Design review of the part built by this model. Coordinates are the model's own, in mm. Face numbers are marked on the shaded views. A direction names the side the tool comes from. Coordinates: 2 decimals unless noted, no trailing zeros. Loops run counter-clockwise (first coordinate to the right, second up) from the corner with the lowest first, then second, coordinate; pieces in that order, holes last. Notation, with made-up numbers: M -39.5,15.5 L -7.5,15.5 A20 cw -7.5,39.5 Z; hole C 26.5,44.5 d11. An arc over 180 degrees is marked long. One line per item, written item: value.
```python
from build123d import *

# Parameters (mm, degrees)
F1_DEPTH  = 25
F3_DEPTH  = 3.96875
F4_R      = 3.81
F5_DEPTH  = 21.001
F6_R      = 7.5
F7_DEPTH  = 2
F8_R      = 26.5
F8_R_2    = 21.5
F9_DEPTH  = 25
F10_W     = 41.7897145033
F10_H     = 10
F11_DEPTH = 26.501
F12_R     = 5
F13_R     = 12


# Not quite as in the source:
# - a length typed as a fraction of an inch, garbled in the dataset ("3 / 203.2 mm" for 3/8 in), is restored


with BuildPart() as f1:
    # F0 (on Right) → F1 (new body, symmetric)
    with BuildSketch(Plane.YZ):
        with BuildLine():
            Line((-24.2330926563, 5), (-9.2330926563, 5))
            ThreePointArc((-9.2330926563, 5), (-5.3735463151, 9.0208092763), (0, 10.5))
            Line((0, 10.5), (-24.2330926563, 10.5))
            Line((-24.2330926563, 10.5), (-24.2330926563, 5))
        make_face()
        with BuildLine():
            ThreePointArc((-2.2912878475, 5), (2.9705148408, 4.628827236), (5.5, 0))
            ThreePointArc((5.5, 0), (2.9705148408, -4.628827236), (-2.2912878475, -5))
            Line((-2.2912878475, -5), (-9.2330926563, -5))
            ThreePointArc((-9.2330926563, -5), (-5.3735463151, -9.0208092763), (0, -10.5))
            ThreePointArc((0, -10.5), (7.4246212025, -7.4246212025), (10.5, 0))
            ThreePointArc((10.5, 0), (7.4246212025, 7.4246212025), (0, 10.5))
            ThreePointArc((0, 10.5), (-5.3735463151, 9.0208092763), (-9.2330926563, 5))
            Line((-9.2330926563, 5), (-2.2912878475, 5))
        make_face()
        with BuildLine():
            ThreePointArc((0, -10.5), (-5.3735463151, -9.0208092763), (-9.2330926563, -5))
            Line((-9.2330926563, -5), (-24.2330926563, -5))
            Line((-24.2330926563, -5), (-24.2330926563, -10.5))
            Line((-24.2330926563, -10.5), (0, -10.5))
        make_face()
    extrude(amount=F1_DEPTH, both=True)

    # F2 (on face) → F3 (cut)
    with BuildSketch(Plane(origin=(0, 0, -10.5), x_dir=(1, 0, 0), z_dir=(0, 0, -1))):
        Polygon((19.1395280957, 12.1165463282), (15.8197640478, 17.8665463282), (9.1802359522, 17.8665463282), (5.8604719043, 12.1165463282), (9.1802359522, 6.3665463282), (15.8197640478, 6.3665463282), align=None)
        Polygon((-15.8197640478, 6.3665463282), (-9.1802359522, 6.3665463282), (-5.8604719043, 12.1165463282), (-9.1802359522, 17.8665463282), (-15.8197640478, 17.8665463282), (-19.1395280957, 12.1165463282), align=None)
    extrude(amount=-F3_DEPTH, mode=Mode.SUBTRACT)

    # F4 (on face) → F5 (cut, through all)
    with BuildSketch(Plane(origin=(0, 0, -10.5), x_dir=(1, 0, 0), z_dir=(0, 0, -1))):
        with Locations((12.5, 12.1165463282)):
            Circle(F4_R)
        with Locations((-12.5, 12.1165463282)):
            Circle(F4_R)
    extrude(amount=-F5_DEPTH, mode=Mode.SUBTRACT)

    # F6 (on face) → F7 (cut)
    with BuildSketch(Plane.XY.offset(10.5)):
        with Locations((-12.5, -12.1165463282)):
            Circle(F6_R)
        with Locations((12.5, -12.1165463282)):
            Circle(F6_R)
    extrude(amount=-F7_DEPTH, mode=Mode.SUBTRACT)

    # F8 (on Right) → F9 (join, symmetric)
    with BuildSketch(Plane.YZ):
        with Locations((32, 0)):
            Circle(F8_R)
        with Locations((32, 0)):
            Circle(F8_R_2, mode=Mode.SUBTRACT)
    extrude(amount=F9_DEPTH, both=True)

    # F10 (on Top) → F11 (cut, through all)
    with BuildSketch(Plane.XY):
        with Locations((25.8948572517, 32)):
            Rectangle(F10_W, F10_H)
        with BuildLine():
            ThreePointArc((5, 37), (0, 32), (5, 27))
            Line((5, 27), (5, 37))
        make_face()
    extrude(amount=F11_DEPTH, mode=Mode.SUBTRACT)

    # F12
    f12_edges = [f1.edges().sort_by_distance(p)[0] for p in [
        (25, 27, 23.467276),
        (25, 37, 23.467276),
    ]]
    fillet(f12_edges, radius=F12_R)

    # F13
    f13_edges = [f1.edges().sort_by_distance(p)[0] for p in [
        (0, 6.75, 8.042854),
        (0, 6.75, -8.042854),
    ]]
    fillet(f13_edges, radius=F13_R)


solid = f1.part
```
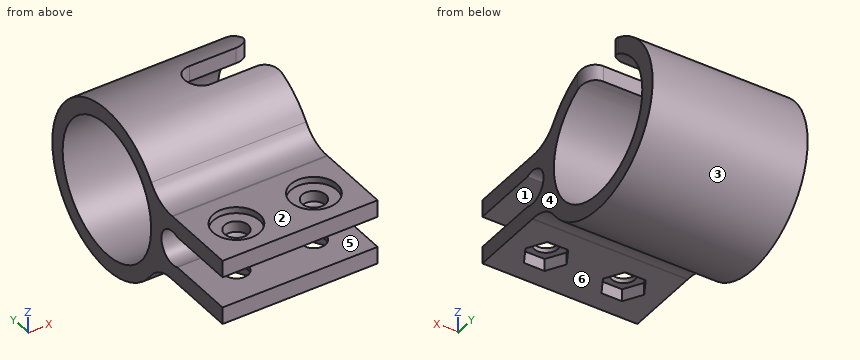
(1) To check wall thickness, follow line 1 along Y through (x, z) = (-19, -8); line 2 along Z through (x, y) = (22.5, -10); line 3 along Y through (x, z) = (18, 10). State the ranges of each line that lie inside material, in increasing order. Write a range as [from, to].
Reply:
line 1: y = [-24.23, -12.36], [-11.87, 12.04], [51.96, 57.26]
line 2: z = [-10.5, -5], [5, 10.5]
line 3: y = [-24.23, -17.22], [-7.02, 12.97], [51.03, 56.54]
(2) Insertion check: pin 1 (10 mm diameter, centred on x = -12.5, y = -12.12, fed in from -Z); pin 2 (6 mm diameter, centred on x = -12.5, y = -12.12, fed in from -Z); pin 3 (24 mm diameter, centred on x = -12.5, y = -12.12, fed in from +Z); pin 4 (3 mm diameter, centred on x = -13.5, z = -8.5, fed in from +Y). Each pin has a flat end and moves straight along its axis. Give the tip position at first contact, or say it passes through.
Reply:
pin 1: stops at z = -6.53
pin 2: passes through
pin 3: stops at z = 10.5
pin 4: stops at y = 57.56
(3) Tool access review of the marked faces 1, 2 and 3: name each direction out of +Z, -Z, +X, -X, +Y, -Y from which nothing blocks a thin tool from reaching the whole face with its end or side.
Reply:
face 1: +X, -X, -Y
face 2: +Z, +X, -X, -Y
face 3: +X, -X
(4) We need section C-C on z = 6.5. State the section outline as (x, y) points, then the cut area to 3 significant figures.
Reply:
outline: M -25,-24.23 L 25,-24.23 L 25,11.51 L -25,11.51 Z; M -25,52.49 L 25,52.49 L 25,57.69 L -25,57.69 Z; hole C -12.5,-12.12 d7.62; hole C 12.5,-12.12 d7.62
area: 1,960 mm2
(5) We need section D-D on x = -12.5. State how many separate pieces and enclosed holes the cut face has, then the cut area to 3 significant figures.
Reply:
separate pieces: 3
enclosed holes: 1
area: 1,000 mm2
(6) We need section A-A on z = 0. State the section outline as (x, y) points, then the cut area to 3 significant figures.
Reply:
outline: M -25,5.5 L 25,5.5 L 25,10.5 L -25,10.5 Z; M -25,53.5 L 25,53.5 L 25,58.5 L -25,58.5 Z
area: 500 mm2
(7) Mouldability with a two-part tool opening along Z and no side actions: class the marked faces 4, 5 and 6 as released by +Z, released by -Z, zero draft, split by the parting line, or undercut.
Reply:
face 4: zero draft
face 5: undercut
face 6: released by -Z
(8) We need section B-B on y = 32. State the section outline as (x, z) points.
Reply:
outline: M -25,-26.5 L 25,-26.5 L 25,-21.5 L -25,-21.5 Z; M -25,21.5 L 0,21.5 L 0,26.5 L -25,26.5 Z
